Source: three-view drawing plus pictorial views. Frame: mm from the lowest corner of the part. A direction names the side the tool comes from. Round coordinates to 2 decimals unless told otherwise and drop trailing zeros. Order: outer loops, then holes, each group sorted by start corner. A loop starts at its lowest first (then second) coordinate and runs counter-clockwise, first axis right, second up. Notation, with made-up numbers: M 6,35 L 39,35 A37 cw 39,73 Z; hole C -28,83.25 d4. An arc over 180 degrees is marked long. Return JSON: item names as keys, results as strings. Group by question number.
Q1. Cut plane A-A on y = 17.5. Output: boundary loops of the cut face in (x, z), and give its area (3 significant figures).
Q2. Cut plane C-C on z = 46.5. Output: boundary loops of the cut face in (x, y), and give its area (3 significant figures).
Q3. Access query for the marked faces 1 and 2. Directions: +Z, -Z, +X, -X, +Y, -Y. A direction counts if a zero-diameter tool reaches every point of the face in a straight line with its end or side. Return the directions, or none.
Q4. Contact query for flat-ended pins moving along their axis: pin 1 (4 mm diameter, centred on y = 15.5, z = 19.5, fed in from -X); pin 2 (10 mm diameter, centred on x = 9, z = 49.5, fed in from -Y). Output: stop coordinate, or through.
Q5. Ray query, probe 1 along Z at (x, y) = (60, 27.5); probe 2 along Y at (x, z) = (24, 54); probe 3 along Y at (x, z) = (9, 57). Return the intervals inside material, ascending.
Q6. Cut plane D-D on x = 39.5. Output: boundary loops of the cut face in (y, z), and give its area (3 significant figures).
Q7. Cut plane B-B on x = 5.5. Output: boundary loops of the cut face in (y, z).
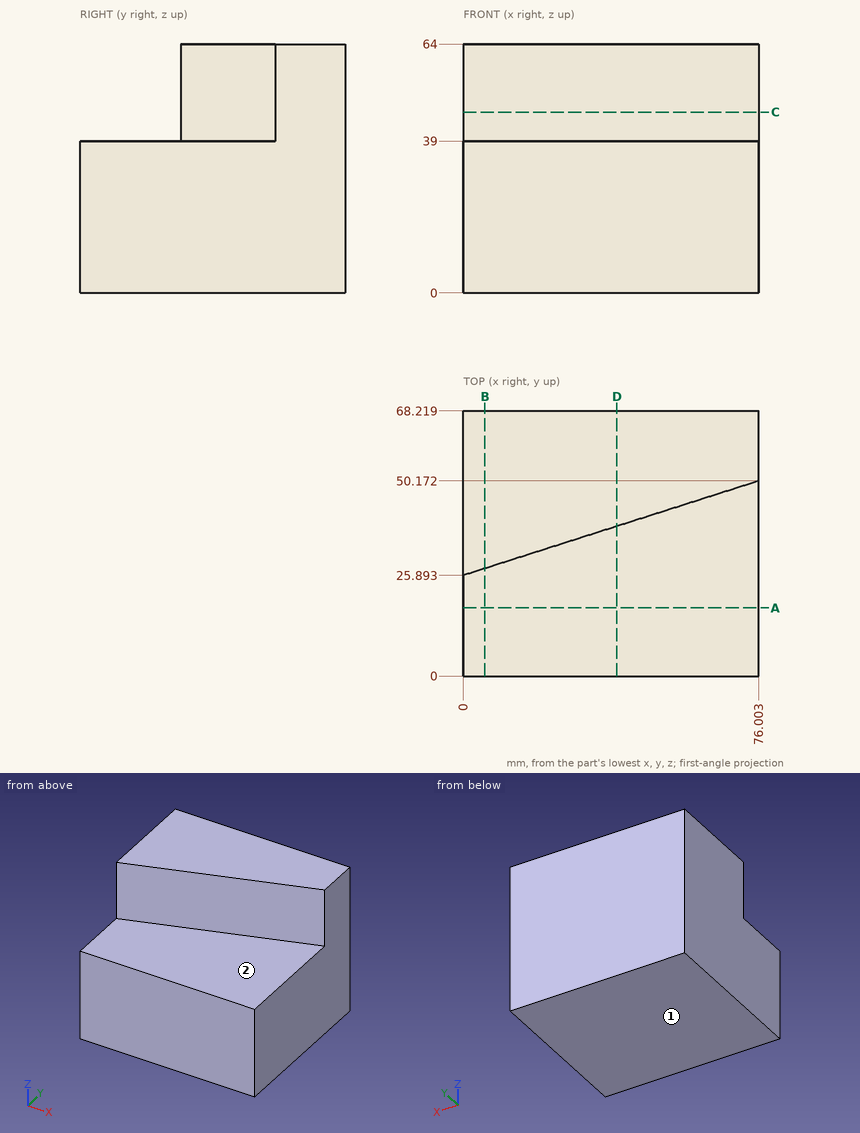
Result sheet:
{
 "1": {"outline": "M 0,0 L 76,0 L 76,39 L 0,39 Z", "area": "2,960 mm²"},
 "2": {"outline": "M 0,25.89 L 76,50.17 L 76,68.22 L 0,68.22 Z", "area": "2,290 mm²"},
 "3": {"face 1": "-Z, +X, -X, +Y, -Y", "face 2": "+Z, +X, -Y"},
 "4": {"pin 1": "stops at x = 0", "pin 2": "stops at y = 27.17"},
 "5": {"probe 1": "z = 0 to 39", "probe 2": "y = 33.56 to 68.22", "probe 3": "y = 28.77 to 68.22"},
 "6": {"outline": "M 0,0 L 68.22,0 L 68.22,64 L 38.51,64 L 38.51,39 L 0,39 Z", "area": "3,400 mm²"},
 "7": {"outline": "M 0,0 L 68.22,0 L 68.22,64 L 27.65,64 L 27.65,39 L 0,39 Z"}
}
